Part print with two shaded views. Sizes in mm from the minimum x, y, z corner. A direction names the side the tool comes from. Give positions to 0.01 mm unless a question says otherwise; leave off trailing zeros. Order: outer loops, then holes, each group sorted by start corner. A loop starts at its lowest first (then second) coordinate and runs counter-clockwise, first axis right, second up. Notation, with made-up numbers: M -0.5,2.5 L 58.5,2.5 A28 ccw 58.5,25.5 Z; hole C 53.5,-5 d4. An arc over 180 degrees is marked long. Return JSON: item names as keys, results as strings.
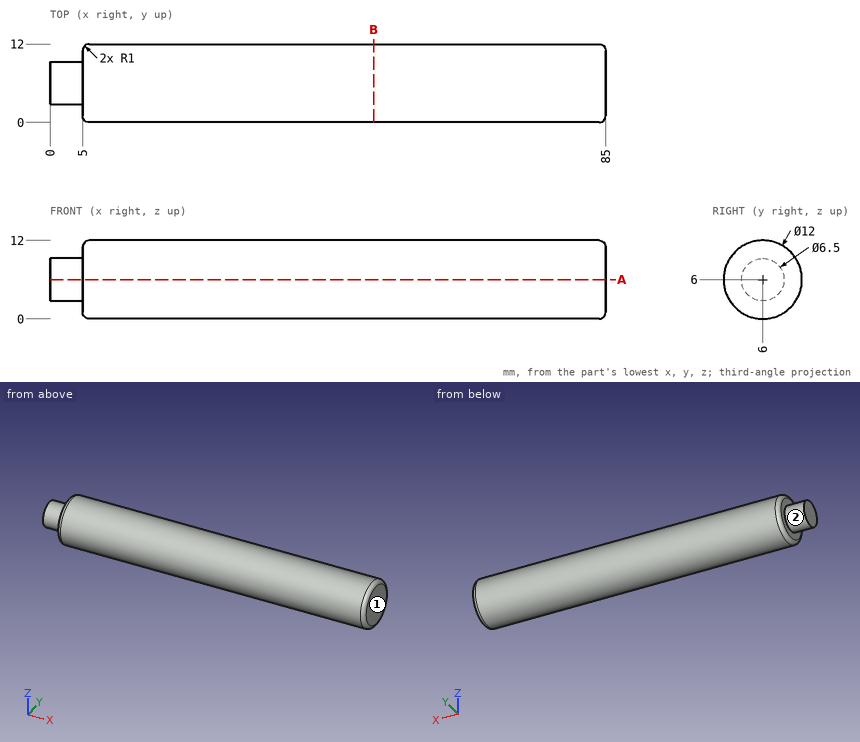
Q1. Probe line 1 along X through (y, z) = (9.75, 8.25); line 2 along Z through (x, y) = (13, 10); line 3 along Y through (x, z) = (13.5, 8). List the from-to ranges inside material, lowest first.
Established:
{"line 1": "x = 5 to 85", "line 2": "z = 1.53 to 10.47", "line 3": "y = 0.34 to 11.66"}
Q2. Band-saw the part on A-A (z = 6). Give the cut face in (x, y), then the cut area to 3 significant figures.
Established:
{"outline": "M 0,2.75 L 5,2.75 L 5,1 A1 ccw 6,0 L 84,0 A1 ccw 85,1 L 85,11 A1 ccw 84,12 L 6,12 A1 ccw 5,11 L 5,9.25 L 0,9.25 Z", "area": "992 mm²"}
Q3. 3-axis set-ups, long thin cutter, end or side, ignore diameter. For the marked faces 1 and 2: which of +Z, -Z, +X, -X, +Y, -Y reach the whole face in a straight line?
Established:
{"face 1": "+Z, -Z, +X, +Y, -Y", "face 2": "-X"}
Q4. Band-saw the part on B-B (x = 49.5). Give the cut face in (y, z), then the cut area to 3 significant figures.
Established:
{"outline": "C 6,6 d12", "area": "113 mm²"}
Q5. Pin check, flat tips, straight feed: pin 1 (1.5 mm diameter, centred on x = 58, y = 4, fed in from +Z); pin 2 (6 mm diameter, centred on x = 37, z = 1.5, fed in from +Y); pin 3 (3 mm diameter, centred on x = 25, y = 2.5, fed in from -Z). Stop position of each tip, or through.
Established:
{"pin 1": "stops at z = 11.87", "pin 2": "stops at y = 11.81", "pin 3": "stops at z = 0.34"}
